For this review, use the dimensioned drawing (mm, ordinates from the lowest corner) and the shaded views. A direction names the side the tool comes from. Coordinates: 2 decimals unless noted, no trailing zeros. Order: outer loops, then holes, each group sorted by start corner. A loop starts at its lowest first (then second) coordinate and runs counter-clockwise, first axis right, second up. Notation, with made-up numbers: M 89,-36 L 96,-36 A19 cw 96,-25 Z; hole C 51,-32.75 d9. An arc over 180 degrees is marked long. One line per item, written item: value.
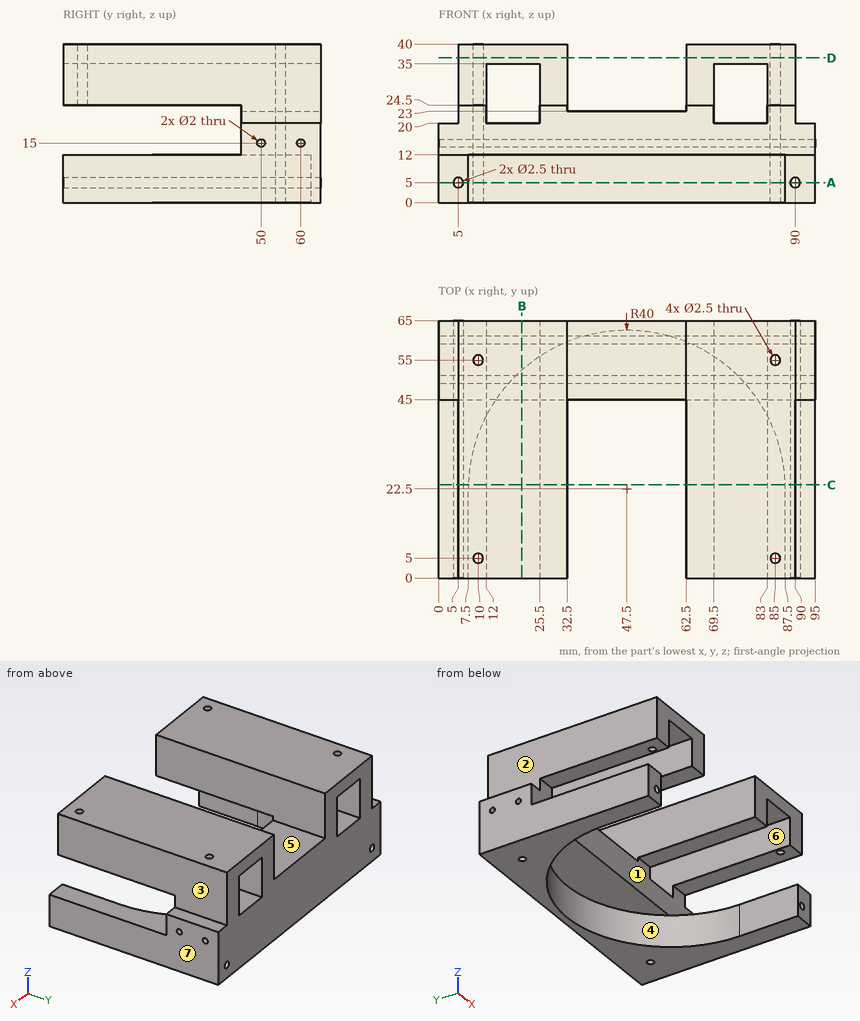
(1) We need section A-A, the plane z = 5. State the section outline as (x, y) points, plus the area to 3 significant figures.
Geometry results:
outline: M 0,0 L 3.75,0 L 3.75,65 L 0,65 Z; M 6.25,0 L 7.5,0 L 7.5,22.5 A40 cw 87.5,22.5 L 87.5,0 L 88.75,0 L 88.75,65 L 6.25,65 Z; M 91.25,0 L 95,0 L 95,65 L 91.25,65 Z; hole C 10,55 d2.5; hole C 85,55 d2.5
area: 1,530 mm2
(2) Mouldability with a two-part tool opening along Z and no side actions: class the marked faces 5, 6 and 7 as +Z half, -Z half, draft (parallel to the pull), parting line (faces both ways), or undercut.
Geometry results:
face 5: +Z half
face 6: undercut
face 7: draft
(3) Insertion check: pin 1 Ø4 at (x, y) = (10, 5) entering from -Z; pin 2 Ø2 at (x, y) = (11, 44.5) entering from -Z; pin 3 Ø10 at (x, z) = (21, 6) entering from -Y; pin 4 Ø13.5 at (y, z) = (28.5, 34) entering from -X. Each pin has a flat end and moves straight along its axis. Give the tip position at first contact, or say it passes through.
Geometry results:
pin 1: stops at z = 24.5
pin 2: stops at z = 0
pin 3: stops at y = 47.15
pin 4: stops at x = 5
(4) Tool access review of the marked faces 1, 2, 3 and 4: name each direction out of +Z, -Z, +X, -X, +Y, -Y from which nothing blocks a thin tool from reaching the whole face with its end or side.
Geometry results:
face 1: +X, -X, -Y
face 2: +Z, -X, +Y, -Y
face 3: +Z, +X, +Y, -Y
face 4: -Z, -Y
(5) We need section D-D, the plane z = 36.5. State the section outline as (x, y) points.
Geometry results:
outline: M 5,0 L 32.5,0 L 32.5,65 L 5,65 Z; M 62.5,0 L 90,0 L 90,65 L 62.5,65 Z; hole C 10,5 d2.5; hole C 10,55 d2.5; hole C 85,5 d2.5; hole C 85,55 d2.5
(6) We need section C-C, the plane y = 23.5. State the section outline as (x, z) points.
Geometry results:
outline: M 0,0 L 7.51,0 L 7.51,12 L 0,12 Z; M 5,24.5 L 12,24.5 L 12,35 L 25.5,35 L 25.5,24.5 L 32.5,24.5 L 32.5,40 L 5,40 Z; M 62.5,24.5 L 69.5,24.5 L 69.5,35 L 83,35 L 83,24.5 L 90,24.5 L 90,40 L 62.5,40 Z; M 87.49,0 L 95,0 L 95,12 L 87.49,12 Z; hole C 5,5 d2.5; hole C 90,5 d2.5
(7) We need section B-B, the plane x = 21. State the section outline as (y, z) points, plus the area to 3 significant figures.
Geometry results:
outline: M 0,35 L 65,35 L 65,40 L 0,40 Z; M 45,12 L 52.46,12 L 52.46,0 L 65,0 L 65,20 L 45,20 Z; hole C 50,15 d2; hole C 60,15 d2
area: 629 mm2
(8) For L1, parallel to Y at x = 25, z = 15; L2, parallel to X at y = 10, z = 36; L3, parallel to X at y = 22, z = 10.5, list the stretches that pass through material, from the lowest coordinate up.
Geometry results:
L1: y = 45 to 49, 51 to 59, 61 to 65
L2: x = 5 to 32.5, 62.5 to 90
L3: x = 0 to 7.5, 87.5 to 95
